Read the model definition and answer for the solid it produces. Units are mm, in the model's axes. A direction names the side the tool comes from. Coordinates: 2 decimals unless noted, no trailing zeros. Write each loop counter-clockwise with the first axis right and the second up, starting at its lowest first coordinate (ties: lowest second). Pieces come first, ordered by that corner, then holes. Notation, with made-up numbers: (84, -33) -> (98, -33) arc R16 cw to (98, -12) -> close; hole circle Ø1 at (42, 68.5). An arc over 180 degrees is marked (long way). Write item = value, one per line. Start each with the question number.
1) Find the intervals of material crossed by line 1 along X through (y, z) = (-1.45, 7.5); line 2 along Z through (x, y) = (0, 1.35); line 3 along Y through (x, z) = (-3, 7.5), in increasing order. Write a range as from..to.
2) Section A-A (y = 1.75) is taken. Determine the outline of the cut face in (x, z).
3) Section B-B (z = 14) is taken. Determine the outline of the cut face in (x, y), plus the area to 3 significant figures.
4) A tool of negligible diameter and unlimited length cuts with its end or side. For faces 1 (the face through (-6, 2, 10)), 2 (the face through (-10, 0, 0)), 3 (the face through (0, -2, 4)), from which of +Z, -Z, +X, -X, +Y, -Y can it reach the whole face along a straight path? Write none if from no direction.
5) Section C-C (x = -4.5) is taken. Determine the outline of the cut face in (y, z), plus the area to 3 significant figures.
6) A flat-ended cylindrical pin translates along its axis: pin 1 Ø3 at (x, z) = (0.5, 12) entering from +Y. Find the tip coordinate at first contact, or state that the pin passes through.
7) For a pull along X with two mould halves and no side action, classify faces 4 (the face through (0, 2, 4)), 5 (the face through (-9.43, 0.04, 19.4)), 6 (the face through (0, 2, 16)), 7 (the face through (0, -2.5, 0)) as released by +X, released by -X, zero draft, split by the parting line, or undercut.
Autodesk Inventor part; units mm, degrees
ref_plane "YZ Plane" through (0, 0, 0) normal (1, 0, 0) x (0, 1, 0)
ref_plane "XZ Plane" through (0, 0, 0) normal (0, 1, 0) x (-1, 0, 0)
ref_plane "XY Plane" through (0, 0, 0) normal (0, 0, 1) x (1, 0, 0)
sketch "草圖1" plane through (0, 0, 0) normal (0, 1, 0) x (-1, 0, 0)
  line L0 (10, 20) -> (-10, 20)
  line L1 (-10, 20) -> (-10, -20)
  line L2 (-10, -20) -> (10, -20)
  line L3 (10, -20) -> (10, 20)
  line L4 (10, 20) -> (-10, -20) construction
  line L5 (-10, 20) -> (10, -20) construction
  point P0 (0, 0)
  dimension "d0" = 20
  dimension "d1" = 40
extrude "擠出1" add sketch "草圖1" along normal mid plane 5
sketch "草圖2" plane through (0, -2.5, 0) normal (0, -1, 0) x (1, 0, 0)
  line L0 (-6, 4) -> (6, 4)
  line L1 (6, 4) -> (6, 16)
  line L2 (6, 16) -> (-6, 16)
  line L3 (-6, 16) -> (-6, 4)
  line L4 (-6, 4) -> (6, 16) construction
  line L5 (6, 4) -> (-6, 16) construction
  line L6 (10, 20) -> (-10, 20)
  point P0 (0, 0)
  point P1 (0, 10)
  point P2 (0, 10)
  dimension "d4" = 12
  dimension "d5" = 12
  dimension "d6" = 10
extrude "擠出2" cut sketch "草圖2" against normal blind 2
fillet "圓角1" radius 2 4 edges at (-10, 0, 20) (10, 0, 20) (10, 0, -20) (-10, 0, -20)
mirror "鏡射1" about plane through (0, 0, 0) normal (0, 1, 0) of "擠出2"
equation "\"d5\" = d4"
properties part number "維修門固定器"
Answer key:
q1.line_1 = -10..-6, 6..10
q1.line_2 = -20..4, 16..20
q1.line_3 = -0.5..0.5
q2.outline = (-10, -18) arc R2 ccw to (-8, -20) -> (8, -20) arc R2 ccw to (10, -18) -> (10, 18) arc R2 ccw to (8, 20) -> (-8, 20) arc R2 ccw to (-10, 18) -> close; hole (-6, 4) -> (6, 4) -> (6, 16) -> (-6, 16) -> close
q3.outline = (-10, -2.5) -> (-6, -2.5) -> (-6, -0.5) -> (6, -0.5) -> (6, -2.5) -> (10, -2.5) -> (10, 2.5) -> (6, 2.5) -> (6, 0.5) -> (-6, 0.5) -> (-6, 2.5) -> (-10, 2.5) -> close
q3.area = 52.0 mm^2
q4.face_1 = +Y
q4.face_2 = +Z, -Z, -X, +Y, -Y
q4.face_3 = -Y
q5.outline = (-2.5, -20) -> (2.5, -20) -> (2.5, 4) -> (0.5, 4) -> (0.5, 16) -> (2.5, 16) -> (2.5, 20) -> (-2.5, 20) -> (-2.5, 16) -> (-0.5, 16) -> (-0.5, 4) -> (-2.5, 4) -> close
q5.area = 152 mm^2
q6.pin_1 = 0.5
q7.face_4 = undercut
q7.face_5 = released by -X
q7.face_6 = undercut
q7.face_7 = zero draft
